Answer from the drawing. Dimensions are ordinates in mm from the lowest x, y and z of the part. A direction names the side the tool comes from. Give positions to 0.01 mm unless a question says otherwise; leave off trailing zeros. Order: outer loops, then holes, each group sorted by start corner. A loop starts at its lowest first (then second) coordinate and runs counter-clockwise, first axis right, second up. Notation, with made-up numbers: (-6, -5) -> (50, -5) arc R26 ccw to (50, 13) -> close; hole circle Ø1 at (30, -21.5). An arc over 180 degrees is marked (long way). Write item = value, one per line. Start each with the question number.
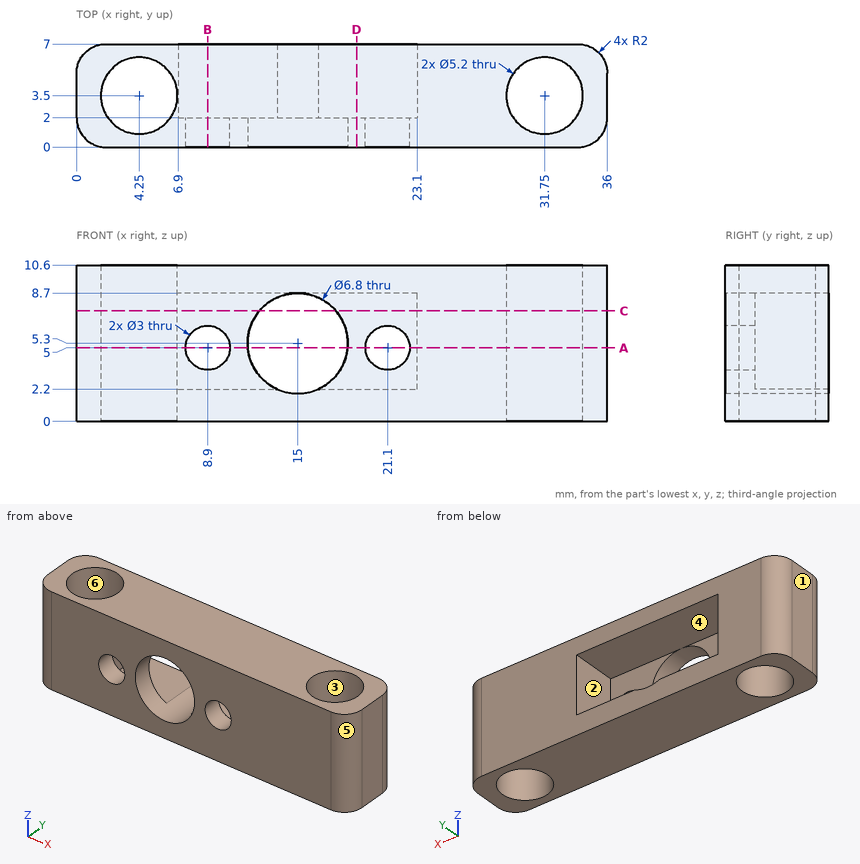
Item 1: A cutting plane is placed at C-C, the plane z = 7.5. Write down the section's boundary in (x, y).
Item 2: A cutting plane is placed at A-A, the plane z = 5. Write down the section's boundary in (x, y), plus the area to 3 significant figures.
Item 3: Which of the six approach directions +Z, -Z, +X, -X, +Y, -Y give full straight-line access (tool end or side, diameter ignored) to the marked faces 1 and 2?
Item 4: Consider L1, parallel to Z at x = 15, y = 1.75; L2, parallel to Y at x = 31.75, z = 4.25; L3, parallel to X at y = 5.5, z = 10.25. Determine where each line is inside the solid, lowest interval first. Write a range as from..to.
Item 5: The mould has two halves that part along Y. Classify the marked faces 3, 4, 5 and 6: +Y half, -Y half, draft (parallel to the pull), parting line (faces both ways), or undercut.
Item 6: A cutting plane is placed at D-D, the plane x = 19. Write down the section's boundary in (y, z), plus the area to 3 significant figures.
Item 7: A cutting plane is placed at B-B, the plane x = 8.9. Write down the section's boundary in (y, z).
Item 8: Flat-ended cylindrical pins translate along their axes: pin 1 (3.5 mm diameter, centred on x = 21.1, z = 5, fed in from +Y); pin 2 (5 mm diameter, centred on x = 10.5, z = 4, fed in from +Y). Find the tip coordinate at first contact, or state that the pin passes through.
Check values:
q1.outline = (0, 2) arc R2 ccw to (2, 0) -> (12.41, 0) -> (12.41, 2) -> (6.9, 2) -> (6.9, 7) -> (2, 7) arc R2 ccw to (0, 5) -> close; (17.59, 0) -> (34, 0) arc R2 ccw to (36, 2) -> (36, 5) arc R2 ccw to (34, 7) -> (23.1, 7) -> (23.1, 2) -> (17.59, 2) -> close; hole circle Ø5.2 at (4.25, 3.5); hole circle Ø5.2 at (31.75, 3.5)
q2.outline = (0, 2) arc R2 ccw to (2, 0) -> (7.4, 0) -> (7.4, 2) -> (6.9, 2) -> (6.9, 7) -> (2, 7) arc R2 ccw to (0, 5) -> close; (10.4, 0) -> (11.61, 0) -> (11.61, 2) -> (10.4, 2) -> close; (18.39, 0) -> (19.6, 0) -> (19.6, 2) -> (18.39, 2) -> close; (22.6, 0) -> (34, 0) arc R2 ccw to (36, 2) -> (36, 5) arc R2 ccw to (34, 7) -> (23.1, 7) -> (23.1, 2) -> (22.6, 2) -> close; hole circle Ø5.2 at (4.25, 3.5); hole circle Ø5.2 at (31.75, 3.5)
q2.area = 99.5 mm^2
q3.face_1 = +Z, -Z, -X, +Y, -Y
q3.face_2 = +Y
q4.L1 = 0..1.9, 8.7..10.6
q4.L2 = 0..0.9, 6.1..7
q4.L3 = 0.06..2.59, 5.91..30.09, 33.41..35.94
q5.face_3 = undercut
q5.face_4 = draft
q5.face_5 = -Y half
q5.face_6 = undercut
q6.outline = (0, 0) -> (7, 0) -> (7, 2.2) -> (2, 2.2) -> (2, 8.7) -> (7, 8.7) -> (7, 10.6) -> (0, 10.6) -> close
q6.area = 41.7 mm^2
q7.outline = (0, 0) -> (7, 0) -> (7, 2.2) -> (2, 2.2) -> (2, 3.5) -> (0, 3.5) -> close; (0, 6.5) -> (2, 6.5) -> (2, 8.7) -> (7, 8.7) -> (7, 10.6) -> (0, 10.6) -> close
q8.pin_1 = 2
q8.pin_2 = 7
